from build123d import *

# Parameters (mm, degrees)
BOSS_EXTRU_1_DEPTH           = 10
ENL_V_MAT_EXTRU_1_DEPTH      = 31.789608707
ENL_V_MAT_EXTRU_1_DEPTH_BACK = 31.789608707
ESQUISSE2_OUTSIDE_W          = 69.818
ESQUISSE2_OUTSIDE_H          = 23.818
ESQUISSE3_R                  = 4
BOSS_EXTRU_2_DEPTH           = 0.3
TROU_TARAUD_M31_D            = 2.5


with BuildPart() as part:
    # Esquisse1 → Boss.-Extru.1 (new body)
    with BuildSketch(Plane(origin=(0, 0, 0), x_dir=(1, 0, 0), z_dir=(0, 1, 0))):
        with BuildLine():
            Line((-20, -7.99999973), (20, -7.99999973))
            ThreePointArc((20, -7.99999973), (26.449806199, 4.732864097), (12.368486389, 2.40000027))
            ThreePointArc((12.368486389, 2.40000027), (11.643823942, 1.38754872), (10.460607986, 1.00000027))
            Line((10.460607986, 1.00000027), (-10.460607986, 1.00000027))
            ThreePointArc((-10.460607986, 1.00000027), (-11.643823942, 1.38754872), (-12.368486389, 2.40000027))
            ThreePointArc((-12.368486389, 2.40000027), (-26.449806199, 4.732864097), (-20, -7.99999973))
        make_face()
    extrude(amount=BOSS_EXTRU_1_DEPTH)

    # Esquisse2 outside → Enlèv. mat.-Extru.1 (cut, two sides: drawn at the far end of the back side and taken through both)
    with BuildSketch(Plane.XY.offset(-ENL_V_MAT_EXTRU_1_DEPTH_BACK)):
        with Locations((0, 5)):
            Rectangle(ESQUISSE2_OUTSIDE_W, ESQUISSE2_OUTSIDE_H)
        with BuildLine():
            Line((7, 10), (-7, 10))
            ThreePointArc((-7, 10), (-9.828427125, 8.828427125), (-11, 6))
            Line((-11, 6), (-11, 4))
            ThreePointArc((-11, 4), (-11.292893219, 3.292893219), (-12, 3))
            Line((-12, 3), (-28, 3))
            Line((-28, 3), (-28, 0))
            Line((-28, 0), (-12, 0))
            ThreePointArc((-12, 0), (-9.171572875, 1.171572875), (-8, 4))
            Line((-8, 4), (-8, 6))
            ThreePointArc((-8, 6), (-7.707106781, 6.707106781), (-7, 7))
            Line((-7, 7), (7, 7))
            ThreePointArc((7, 7), (7.707106781, 6.707106781), (8, 6))
            Line((8, 6), (8, 4))
            ThreePointArc((8, 4), (9.171572875, 1.171572875), (12, 0))
            Line((12, 0), (28, 0))
            Line((28, 0), (28, 3))
            Line((28, 3), (12, 3))
            ThreePointArc((12, 3), (11.292893219, 3.292893219), (11, 4))
            Line((11, 4), (11, 6))
            ThreePointArc((11, 6), (9.828427125, 8.828427125), (7, 10))
        make_face(mode=Mode.SUBTRACT)
    extrude(amount=ENL_V_MAT_EXTRU_1_DEPTH + ENL_V_MAT_EXTRU_1_DEPTH_BACK, mode=Mode.SUBTRACT)

    # Esquisse3 → Boss.-Extru.2 (add)
    with BuildSketch(Plane.XZ):
        with Locations(Location((20, -2.7e-07, 0), (0, 0, 270))):
            Circle(ESQUISSE3_R)
    boss_extru_2 = extrude(amount=BOSS_EXTRU_2_DEPTH)

    # Esquisse4 → Fraisage pour vis à tête fraisée à 6 pans creux M31 (revolve, cut)
    with BuildSketch(Plane(origin=(20, 3, -2.7e-07), x_dir=(0, 0, 1), z_dir=(1, 0, 0))):
        Polygon((0, 0), (0, 3.3), (1.6, 3.3), (1.6, 1.7), (2.9, 0.4), (2.9, 0), align=None)
    fraisage_pour_vis_t_te_frais_e_6_pan = revolve(axis=Axis((20, 9.35, -2.7e-07), (0, -1, 0)), mode=Mode.SUBTRACT)

    # Trou taraudé M31 (through all)
    with Locations(Plane(origin=(0, 10, 0), x_dir=(1, 0, 0), z_dir=(0, 1, 0))):
        with Locations((0, -3.5)):
            Hole(TROU_TARAUD_M31_D / 2)

    # Symétrie1: Boss.-Extru.2, Fraisage pour vis à tête fraisée à 6 pans creux M31 across plane
    add(boss_extru_2.mirror(Plane(origin=(0, 0, 0), x_dir=(0, 0, 1), z_dir=(1, 0, 0))))
    add(fraisage_pour_vis_t_te_frais_e_6_pan.mirror(Plane(origin=(0, 0, 0), x_dir=(0, 0, 1), z_dir=(1, 0, 0))), mode=Mode.SUBTRACT)


solid = part.part
Could you check a few things on this model? Use its own coordinates, in mm. A direction names the side the tool comes from. Round coordinates to 2 decimals unless told otherwise and drop trailing zeros. Write each loop counter-clockwise with the first axis right and the second up, starting at its lowest first coordinate (ties: lowest second). Pieces come first, ordered by that corner, then holes. Notation, with made-up numbers: (36, 76) - (70, 76) arc R11 ccw to (70, 85) - close; hole circle Ø5 at (-5, 33). An arc over 180 degrees is marked (long way). Use a Markdown table: item, result.
Q1. I want a section at C-C (y = 9). List the corners of the cut face in (x, z) for me.
Output values:
| item | result |
|---|---|
| outline | (-9.65, -1) - (9.65, -1) - (9.65, 8) - (-9.65, 8) - close; hole circle Ø2.5 at (0, 3.5) |
Q2. I want a section at A-A (x = 0). List the corners of the cut face in (y, z) for me.
Output values:
| item | result |
|---|---|
| outline | (7, -1) - (10, -1) - (10, 2.25) - (7, 2.25) - close; (7, 4.75) - (10, 4.75) - (10, 8) - (7, 8) - close |
Q3. Thinking about a two-plate mould opening in X: for faces 1 (the flat face through (20, -0.3, -2)), 2 (the cylindrical face through (9.859, 8.797, 3.399)), 3 (the flat face through (0.1, 7.2, -1)), which applies, released by +X, released by -X, zero draft, split by the parting line, or undercut?
Output values:
| item | result |
|---|---|
| face 1 | zero draft |
| face 2 | released by +X |
| face 3 | undercut |
Q4. I want a section at D-D (z = 6.5). List the corners of the cut face in (x, y) for me, plus the area to 3 significant figures.
Output values:
| item | result |
|---|---|
| outline | (-24.66, 0) - (-12, 0) arc R4 ccw to (-8, 4) - (-8, 6) arc R1 cw to (-7, 7) - (7, 7) arc R1 cw to (8, 6) - (8, 4) arc R4 ccw to (12, 0) - (24.66, 0) - (24.66, 3) - (12, 3) arc R1 cw to (11, 4) - (11, 6) arc R4 ccw to (7, 10) - (-7, 10) arc R4 ccw to (-11, 6) - (-11, 4) arc R1 cw to (-12, 3) - (-24.66, 3) - close |
| area | 177 mm2 |
Q5. For pin 1 (3 mm diameter, centred on y = 5.5, z = -4.5, fed in from +X); pin 2 (7 mm diameter, centred on x = -0.5, z = 3.5, fed in from -Y); pin 3 (5 mm diameter, centred on x = -1.5, y = 5.5, fed in from -Z); pin 4 (2 mm diameter, centred on y = 4.5, z = 2.5, fed in from +X), each with a flat end and sliding along its axis, tell me the tip position at first contact or that it passes through.
Output values:
| item | result |
|---|---|
| pin 1 | through |
| pin 2 | y = 7 |
| pin 3 | z = -1 |
| pin 4 | x = 11.13 |
Q6. For faces 4 (the flat face through (20.1, 3, 3.4)), 5 (the cylindrical face through (-22.83, 2.8, -0.63)), 6 (the flat face through (-19.9, 3, 3.4)), 7 (the flat face through (16, 0, 2)), which set-ups out of +Z, -Z, +X, -X, +Y, -Y let a thin tool reach every point of the face, with its end or its side?
Output values:
| item | result |
|---|---|
| face 4 | +Z, -Z, +X, +Y |
| face 5 | +Y |
| face 6 | +Z, -Z, -X, +Y |
| face 7 | -Y |
Q7. Please list where these lines run through material, in increasing order: L1, parallel to Z at x = 20, y = 2.75; L2, parallel to X at y = 2.9, z = 0; L3, parallel to Z at x = 0, y = 8.8.
Output values:
| item | result |
|---|---|
| L1 | -8 to -2.9, 2.9 to 8 |
| L2 | -28 to -22.9, -17.1 to -8.15, 8.15 to 17.1, 22.9 to 28 |
| L3 | -1 to 2.25, 4.75 to 8 |
